Check sheet for the modelled part. Datum: model origin and axes. Units: mm. Face numbers are marked on the shaded views. A direction names the side the tool comes from. Round coordinates to 2 decimals unless told otherwise and drop trailing zeros. Write each loop counter-clockwise with the first axis right and the second up, starting at its lowest first coordinate (ties: lowest second). Pieces come first, ordered by that corner, then holes. Notation, with made-up numbers: (81.5, -12) -> (140.5, -12) arc R21 ccw to (140.5, -1) -> close; hole circle Ø9 at (18, 21). An arc over 180 degrees is marked (long way). One line per item, written item: value.
from build123d import *

# Parameters (mm, degrees)
F1_DEPTH = 10
F2_R     = 1.25
F3_DEPTH = 1.201
F4_R     = 1
F5_R     = 3


with BuildPart() as f1:
    # F0 (on Front) → F1 (new body)
    with BuildSketch(Plane.XZ):
        with BuildLine():
            ThreePointArc((-1.725, 1.725), (0, 3.45), (1.725, 1.725))
            Line((1.725, 1.725), (1.725, 0))
            Line((1.725, 0), (2.925, 0))
            Line((2.925, 0), (12.925, 0))
            Line((12.925, 0), (12.925, 1.2))
            Line((12.925, 1.2), (2.925, 1.2))
            Line((2.925, 1.2), (2.925, 1.725))
            ThreePointArc((2.925, 1.725), (0, 4.65), (-2.925, 1.725))
            Line((-2.925, 1.725), (-2.925, 1.2))
            Line((-2.925, 1.2), (-12.925, 1.2))
            Line((-12.925, 1.2), (-12.925, 0))
            Line((-12.925, 0), (-2.925, 0))
            Line((-2.925, 0), (-1.725, 0))
            Line((-1.725, 0), (-1.725, 1.725))
        make_face()
    extrude(amount=F1_DEPTH)

    # F2 (on face) → F3 (cut, through all)
    with BuildSketch(Plane.XY.offset(1.2)):
        with Locations((7.925, -5)):
            Circle(F2_R)
        with Locations((-7.925, -5)):
            Circle(F2_R)
    extrude(amount=-F3_DEPTH, mode=Mode.SUBTRACT)

    # F4
    f4_edges = [f1.edges().sort_by_distance(p)[0] for p in [
        (12.925, -10, 0.6),
        (-12.925, -10, 0.6),
        (12.925, 0, 0.6),
        (-12.925, 0, 0.6),
    ]]
    fillet(f4_edges, radius=F4_R)

    # F5
    f5_edges = [f1.edges().sort_by_distance(p)[0] for p in [
        (2.925, -5, 1.2),
        (-2.925, -5, 1.2),
    ]]
    fillet(f5_edges, radius=F5_R)


solid = f1.part
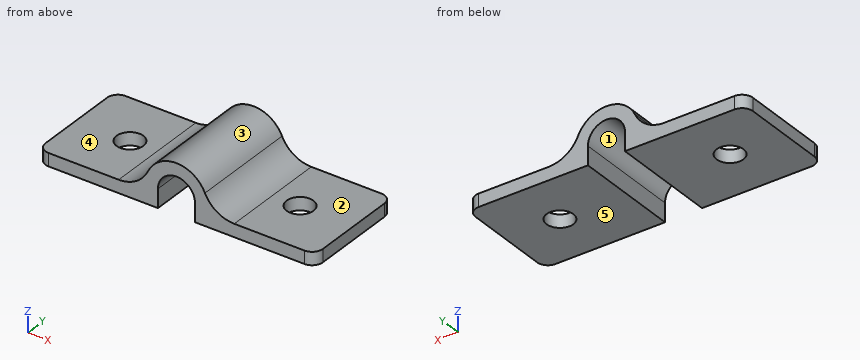
Item 1: Sectioned sample at C-C (x = -7.5). Enter the section's corners in (y, z).
Result set:
outline: (-10, 0) -> (-6.18, 0) -> (-6.18, 1.2) -> (-10, 1.2) -> close; (-3.82, 0) -> (0, 0) -> (0, 1.2) -> (-3.82, 1.2) -> close
Item 2: Material ranges on line 1 along Z through (x, y) = (0, -8.5); line 2 along X through (y, z) = (-7, 2.8); line 3 along Z through (x, y) = (9.75, -6), recorded low to high.
Result set:
line 1: 3.45 to 4.65
line 2: -2.73 to -1.35, 1.35 to 2.73
line 3: 0 to 1.2
Item 3: Tool access check on the marked faces 4 and 5. Record the directions out of +Z, -Z, +X, -X, +Y, -Y that give a thin tool (end or side, any length) a straight path to the whole face; none if there is none.
Result set:
face 4: +Z, -X, +Y, -Y
face 5: -Z, +X, -X, +Y, -Y
Item 4: Depth check by flat-ended pin: pin 1 (2.5 mm diameter, centred on x = -9, y = -5.5, fed in from +Z); pin 2 (1.5 mm diameter, centred on y = -4, z = 2.5, fed in from +X). Enter the tip coordinate at first touch or a pass-through.
Result set:
pin 1: z = 1.2
pin 2: x = 3.65
Item 5: Sectioned sample at B-B (y = -5). State how many separate pieces and enclosed holes the cut face has, then the cut area to 3 significant figures.
Result set:
separate pieces: 3
enclosed holes: 0
area: 32.9 mm^2
Item 6: Sectioned sample at D-D (x = 0). Enter the section's corners in (y, z).
Result set:
outline: (-10, 3.45) -> (0, 3.45) -> (0, 4.65) -> (-10, 4.65) -> close
Item 7: Sectioned sample at A-A (x = 8.75). Enter the section's corners in (y, z).
Result set:
outline: (-10, 0) -> (-5.94, 0) -> (-5.94, 1.2) -> (-10, 1.2) -> close; (-4.06, 0) -> (0, 0) -> (0, 1.2) -> (-4.06, 1.2) -> close
Item 8: Release check for a two-part mould opening along X. For the marked faces 1, 2 and 3 record: pulls with the +X half, pulls with the -X half, needs draft (parallel to the pull), parting line crosses it, or undercut.
Result set:
face 1: undercut
face 2: needs draft
face 3: parting line crosses it
